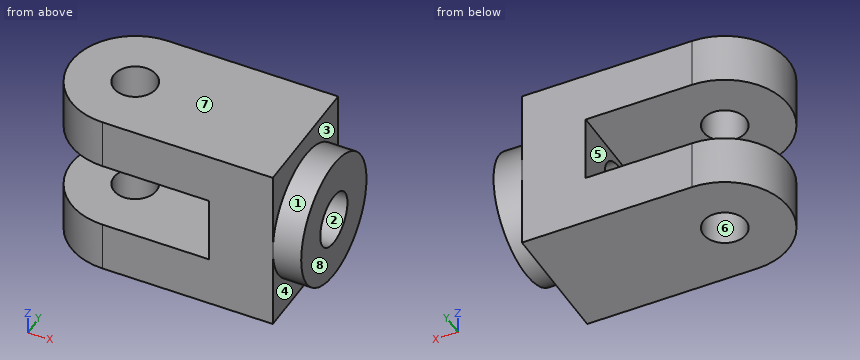
from build123d import *

# Parameters (mm, degrees)
SKETCH1_W               = 132
SKETCH1_H               = 72
BOSS_EXTRUDE1_DEPTH     = 47.625
CUT_EXTRUDE1_DEPTH      = 122.344808294
CUT_EXTRUDE1_DEPTH_BACK = 122.344808294
SKETCH3_W               = 96
SKETCH3_H               = 38.1
CUT_EXTRUDE2_DEPTH      = 85.25
SKETCH4_R               = 15
CUT_EXTRUDE3_DEPTH      = 85.25
BOSS_EXTRUDE2_START     = 16
SKETCH5_R               = 36
SKETCH5_R_2             = 15
BOSS_EXTRUDE2_DEPTH     = 16
CUT_EXTRUDE4_DEPTH      = 131.738527221
CUT_EXTRUDE4_DEPTH_BACK = 131.738527221
SKETCH6_R               = 12
SCALE1_SCALE            = 0.53
SCALE2_SCALE            = 0.66


with BuildPart() as part:
    # Sketch1 → Boss-Extrude1 (new, symmetric)
    with BuildSketch(Plane.XY):
        Rectangle(SKETCH1_W, SKETCH1_H)
    extrude(amount=BOSS_EXTRUDE1_DEPTH, both=True)

    # Sketch2 → Cut-Extrude1 (cut, two sides: drawn at the far end of the back side and taken through both)
    with BuildSketch(Plane.XY.offset(47.625).offset(-CUT_EXTRUDE1_DEPTH_BACK)):
        with BuildLine():
            Line((220.000003209, 36), (-30, 36))
            ThreePointArc((-30, 36), (-66, 1.003e-06), (-30.000002006, -36))
            Line((-30.000002006, -36), (220.000001203, -36.000013927))
            Line((220.000001203, -36.000013927), (-280.000005214, -36))
            Line((-280.000005214, -36), (-280.000003209, 36.000013927))
            Line((-280.000003209, 36.000013927), (220.000003209, 36))
        make_face()
    extrude(amount=CUT_EXTRUDE1_DEPTH + CUT_EXTRUDE1_DEPTH_BACK, mode=Mode.SUBTRACT)

    # Sketch3 → Cut-Extrude2 (cut)
    with BuildSketch(Plane(origin=(0, 36, 0), x_dir=(1, 0, 0), z_dir=(0, 1, 0))):
        with Locations((-18, 0)):
            Rectangle(SKETCH3_W, SKETCH3_H)
    extrude(amount=-CUT_EXTRUDE2_DEPTH, mode=Mode.SUBTRACT)

    # Sketch4 → Cut-Extrude3 (cut)
    with BuildSketch(Plane(origin=(66, 0, 0), x_dir=(0, 0, -1), z_dir=(1, 0, 0))):
        with Locations(Location((0, 0, 0), (0, 0, 90))):
            Circle(SKETCH4_R)
    extrude(amount=-CUT_EXTRUDE3_DEPTH, mode=Mode.SUBTRACT)

    # Sketch5 → Boss-Extrude2 (add)
    with BuildSketch(Plane(origin=(66, 0, 0), x_dir=(0, 0, -1), z_dir=(1, 0, 0)).offset(BOSS_EXTRUDE2_START)):
        with Locations(Location((0, 0, 0), (0, 0, 90))):
            Circle(SKETCH5_R)
        with Locations(Location((0, 0, 0), (0, 0, 90))):
            Circle(SKETCH5_R_2, mode=Mode.SUBTRACT)
    extrude(amount=-BOSS_EXTRUDE2_DEPTH)

    # Sketch6 → Cut-Extrude4 (cut, two sides: drawn at the far end of the back side and taken through both)
    with BuildSketch(Plane.XY.offset(47.625).offset(-CUT_EXTRUDE4_DEPTH_BACK)):
        with Locations((-30, 0)):
            Circle(SKETCH6_R)
    extrude(amount=CUT_EXTRUDE4_DEPTH + CUT_EXTRUDE4_DEPTH_BACK, mode=Mode.SUBTRACT)


with BuildPart() as part_1:
    # Scale1: scaled about (16.519385086, 0, 0)
    add(part.part.scale(SCALE1_SCALE).moved(Location((7.76411099, 0, 0))))


with BuildPart() as part_2:
    # Scale2: scaled about (16.519385086, 0, 0)
    add(part_1.part.scale(SCALE2_SCALE).moved(Location((5.616590929, 0, 0))))


solid = part_2.part
The listing builds one solid part. Answer for the finished solid, in the listing's coordinates (mm). Face numbers are marked on the shaded views. A direction names the side the tool comes from. Coordinates: 2 decimals unless noted, no trailing zeros. Write each loop counter-clockwise with the first axis right and the second up, starting at its lowest first coordinate (ties: lowest second). Pieces come first, ordered by that corner, then holes. Notation, with made-up numbers: (17.5, 29) -> (48.5, 29) arc R19 cw to (48.5, 53) -> close; hole circle Ø5 at (19, 76.5). An arc over 180 degrees is marked (long way). One line per question, with ' | ' between items.
1. Section D-D (y = -7) is taken. Determine the outline of the cut face in (x, z), and give its area (3 significant figures).
Verdict:
outline: (-10.22, -16.66) -> (33.83, -16.66) -> (33.83, -10.47) -> (39.42, -10.47) -> (39.42, 10.47) -> (33.83, 10.47) -> (33.83, 16.66) -> (-10.22, 16.66) -> (-10.22, 6.66) -> (21.23, 6.66) -> (21.23, -6.66) -> (-10.22, -6.66) -> close | area: 1,170 mm^2
2. Section C-C (x = 30) is taken. Determine the outline of the cut face in (y, z), and give its area (3 significant figures).
Verdict:
outline: (-12.59, -16.66) -> (12.59, -16.66) -> (12.59, 16.66) -> (-12.59, 16.66) -> close; hole circle Ø10.49 at (0, 0) | area: 753 mm^2
3. For a pull along X with two mould halves and no side action, classify the marked faces 6, 7 and 8 as released by +X, released by -X, zero draft, split by the parting line, or undercut.
Verdict:
face 6: undercut | face 7: zero draft | face 8: released by +X
4. Section B-B (y = 0) is taken. Determine the outline of the cut face in (x, z).
Verdict:
outline: (-12.35, -16.66) -> (-3.95, -16.66) -> (-3.95, -6.66) -> (-12.35, -6.66) -> close; (-12.35, 6.66) -> (-3.95, 6.66) -> (-3.95, 16.66) -> (-12.35, 16.66) -> close; (4.44, -16.66) -> (33.83, -16.66) -> (33.83, -12.59) -> (39.42, -12.59) -> (39.42, -5.25) -> (21.23, -5.25) -> (21.23, -6.66) -> (4.44, -6.66) -> close; (4.44, 6.66) -> (21.23, 6.66) -> (21.23, 5.25) -> (39.42, 5.25) -> (39.42, 12.59) -> (33.83, 12.59) -> (33.83, 16.66) -> (4.44, 16.66) -> close
5. Straight lines are drawn through the part: line 1 (Z direction, x = 29.5, y = 0); line 2 (X direction, y = 0.25, z = -14); line 3 (Z direction, x = 17, y = 4.5). For each, find the intervals that lie inside material, in ascending order.
Verdict:
line 1: z = -16.66 to -5.25, 5.25 to 16.66 | line 2: x = -12.34 to -3.94, 4.44 to 33.83 | line 3: z = -16.66 to -6.66, 6.66 to 16.66
6. Given pin 1 Ø5 at (x, z) = (1.5, 6) entering from +Y; pin 2 Ø8.5 at (y, z) = (0, 0) entering from -X; pin 3 Ø6.5 at (y, z) = (3.5, -2) entering from -X, each flat-ended and moving along its own axis, determine where each tip first touches the part or whether it passes through.
Verdict:
pin 1: stops at y = 12.59 | pin 2: passes through | pin 3: stops at x = 21.23
7. Section A-A (x = 13.5) is taken. Determine the outline of the cut face in (y, z), and give its area (3 significant figures).
Verdict:
outline: (-12.59, -16.66) -> (12.59, -16.66) -> (12.59, -6.66) -> (-12.59, -6.66) -> close; (-12.59, 6.66) -> (12.59, 6.66) -> (12.59, 16.66) -> (-12.59, 16.66) -> close | area: 503 mm^2
8. Which of the six approach directions +Z, -Z, +X, -X, +Y, -Y give full straight-line access (tool end or side, diameter ignored) to the marked faces 1, 2, 3, 4 and 5?
Verdict:
face 1: +X | face 2: +X, -X | face 3: +Z, +X | face 4: -Z, +X | face 5: -X, +Y, -Y
